The listing builds one solid part. Answer for the finished solid, in the listing's coordinates (mm). Face numbers are marked on the shaded views. Coordinates: 2 decimals unless noted, no trailing zeros. Order: outer loops, then holes, each group sorted by start corner. A loop starts at its lowest first (then second) coordinate and runs counter-clockwise, first axis right, second up. Notation, with made-up numbers: (77, -28.5) -> (133, -28.5) arc R36 cw to (133, 5.5) -> close; hole circle Ø1 at (51, 69.25). An arc over 180 degrees is marked (long way). One line per question, with ' | ' between items.
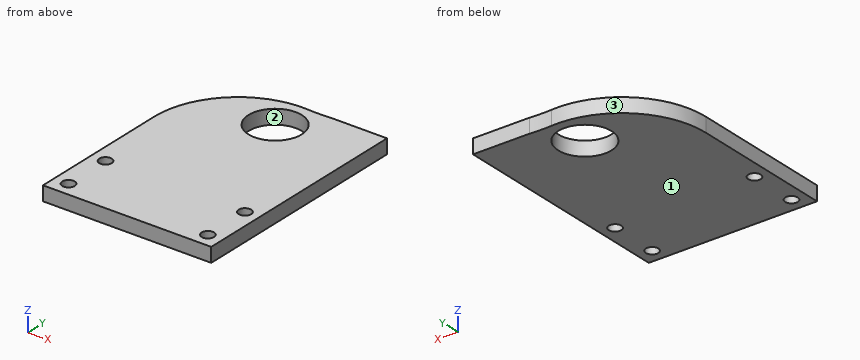
from build123d import *

# Parameters (mm, degrees)
IZIM1_R                     = 11.075
IZIM1_R_2                   = 2.6
Y_KSEKLIK_EKSTR_ZYON1_DEPTH = 6
IZIM2_W                     = 40.176949225
IZIM2_H                     = 32.938980449
Y_KSEKLIK_EKSTR_ZYON2_DEPTH = 6
IZIM3_W                     = 23.482339904
IZIM3_H                     = 35
Y_KSEKLIK_EKSTR_ZYON3_DEPTH = 6
RADYUS1_R                   = 60


with BuildPart() as part:
    # Çizim1 → Yükseklik-Ekstrüzyon1 (new body)
    with BuildSketch(Plane.XY):
        with BuildLine():
            Line((-56.410377678, 29.652139902), (-56.410377678, -30.347860098))
            Line((-56.410377678, -30.347860098), (13.589622322, -30.347860098))
            Line((13.589622322, -30.347860098), (13.589622322, 29.652139902))
            ThreePointArc((13.589622322, 29.652139902), (-21.410377678, 64.652139902), (-56.410377678, 29.652139902))
        make_face()
        with Locations((-21.410377678, 49.652139902)):
            Circle(IZIM1_R, mode=Mode.SUBTRACT)
        with Locations((-50.410377678, -24.347860098)):
            Circle(IZIM1_R_2, mode=Mode.SUBTRACT)
        with Locations((7.589622322, -24.347860098)):
            Circle(IZIM1_R_2, mode=Mode.SUBTRACT)
        with Locations((-50.410377678, -4.347860098)):
            Circle(IZIM1_R_2, mode=Mode.SUBTRACT)
        with Locations((7.589622322, -4.347860098)):
            Circle(IZIM1_R_2, mode=Mode.SUBTRACT)
        with BuildLine():
            Line((-12.410377678, 4.652139902), (-12.410377678, -5.347860098))
            ThreePointArc((-12.410377678, -5.347860098), (-21.410377678, -14.347860098), (-30.410377678, -5.347860098))
            Line((-30.410377678, -5.347860098), (-30.410377678, 4.652139902))
            ThreePointArc((-30.410377678, 4.652139902), (-21.410377678, 13.652139902), (-12.410377678, 4.652139902))
        make_face(mode=Mode.SUBTRACT)
        with BuildLine():
            Line((-33.810377678, 4.652139902), (-33.810377678, -5.347860098))
            ThreePointArc((-33.810377678, -5.347860098), (-35.910377678, -7.447860098), (-38.010377678, -5.347860098))
            Line((-38.010377678, -5.347860098), (-38.010377678, 4.652139902))
            ThreePointArc((-38.010377678, 4.652139902), (-35.910377678, 6.752139902), (-33.810377678, 4.652139902))
        make_face(mode=Mode.SUBTRACT)
        with BuildLine():
            Line((-4.810377678, 4.652139902), (-4.810377678, -5.347860098))
            ThreePointArc((-4.810377678, -5.347860098), (-6.910377678, -7.447860098), (-9.010377678, -5.347860098))
            Line((-9.010377678, -5.347860098), (-9.010377678, 4.652139902))
            ThreePointArc((-9.010377678, 4.652139902), (-6.910377678, 6.752139902), (-4.810377678, 4.652139902))
        make_face(mode=Mode.SUBTRACT)
    extrude(amount=Y_KSEKLIK_EKSTR_ZYON1_DEPTH)

    # Çizim2 → Yükseklik-Ekstrüzyon2 (add)
    with BuildSketch(Plane(origin=(0, 0, 0), x_dir=(-1, 0, 0), z_dir=(0, 0, -1))):
        with Locations((20.088474613, 1.726881697)):
            Rectangle(IZIM2_W, IZIM2_H)
    extrude(amount=-Y_KSEKLIK_EKSTR_ZYON2_DEPTH)

    # Çizim3 → Yükseklik-Ekstrüzyon3 (add)
    with BuildSketch(Plane(origin=(0, 0, 0), x_dir=(-1, 0, 0), z_dir=(0, 0, -1))):
        with Locations((-1.84845237, 47.152139902)):
            Rectangle(IZIM3_W, IZIM3_H)
    extrude(amount=-Y_KSEKLIK_EKSTR_ZYON3_DEPTH)

    # Radyus1
    # the kernel refuses this fillet: 60 mm, written as the material it adds along each edge
    with BuildSketch(Plane(origin=(-9.892717582, 62.702760258, 6), x_dir=(0, 1, 0), z_dir=(0, 0, -1))) as radyus1_piece_1:
        with BuildLine():
            CenterArc((61.73230625, -5.099184882), RADYUS1_R, 175.124756337, 8.749263652)
            Line((1.869405236, -9.152958702), (0.672147215, -9.234034178))
            ThreePointArc((0.672147215, -9.234034178), (0.065725416, -4.753959725), (-1.133164126, -0.394891203))
            Line((-1.133164126, -0.394891203), (0, 1.2))
            ThreePointArc((0, 1.2), (0.974689822, 1.2), (0.753721112, 0.101983698))
            Line((0.753721112, 0.101983698), (1.949379644, 0))
        make_face()
    extrude(amount=6)


solid = part.part
Item 1: Section B-B, the plane y = 55.5 is taken. Give the vertices of the cut face in (x, z).
Computed values:
outline: (-45.01, 0) -> (-30.82, 0) -> (-30.82, 6) -> (-45.01, 6) -> close; (-12.01, 0) -> (13.59, 0) -> (13.59, 6) -> (-12.01, 6) -> close
Item 2: Find the intervals of material crossed by L1, parallel to Y at x = 8.5, z = 2; L2, parallel to Y at x = -21, z = 1.55; L3, parallel to Y at x = -48.5, z = 1.5, in increasing order.
Computed values:
L1: y = -30.35 to -26.78, -21.91 to -6.78, -1.91 to 64.65 | L2: y = -30.35 to 38.58, 60.72 to 64.65 | L3: y = -30.35 to -26.11, -22.58 to -6.11, -2.58 to 51.81
Item 3: Section C-C, the plane z = 4.7 is taken. Give the vertices of the cut face in (x, y) (3 decimals), plus the area to 3 significant figures.
Computed values:
outline: (-56.41, -30.348) -> (13.59, -30.348) -> (13.59, 64.652) -> (-9.893, 64.652) arc R60 cw to (-19.046, 64.572) arc R35 ccw to (-56.41, 29.652) -> close; hole circle Ø5.2 at (-50.41, -24.348); hole circle Ø5.2 at (-50.41, -4.348); hole circle Ø22.15 at (-21.41, 49.652); hole circle Ø5.2 at (7.59, -24.348); hole circle Ø5.2 at (7.59, -4.348) | area: 5,920 mm^2
Item 4: Determine the mould class of the marked faces 1, 2 and 3 for opening direction Y: pulls with the +Y half, pulls with the -Y half, needs draft (parallel to the pull), parting line crosses it, or undercut.
Computed values:
face 1: needs draft | face 2: undercut | face 3: pulls with the +Y half
Item 5: Section A-A, the plane x = -18 is taken. Give the vertices of the cut face in (y, z), plus the area to 3 significant figures.
Computed values:
outline: (-30.35, 0) -> (39.12, 0) -> (39.12, 6) -> (-30.35, 6) -> close; (60.19, 0) -> (64.51, 0) -> (64.51, 6) -> (60.19, 6) -> close | area: 443 mm^2
Item 6: This flat-tipped pin is pushed along its axis until it touches: pin 1 Ø4.5 at (x, y) = (7.59, -24.35) entering from +Z. Where does it stop, or does it pass through?
Computed values:
pin 1: passes through
Item 7: Section D-D, the plane x = 7.5 is taken. Give the vertices of the cut face in (y, z), plus the area to 3 significant figures.
Computed values:
outline: (-30.35, 0) -> (-26.95, 0) -> (-26.95, 6) -> (-30.35, 6) -> close; (-21.75, 0) -> (-6.95, 0) -> (-6.95, 6) -> (-21.75, 6) -> close; (-1.75, 0) -> (64.65, 0) -> (64.65, 6) -> (-1.75, 6) -> close | area: 508 mm^2
